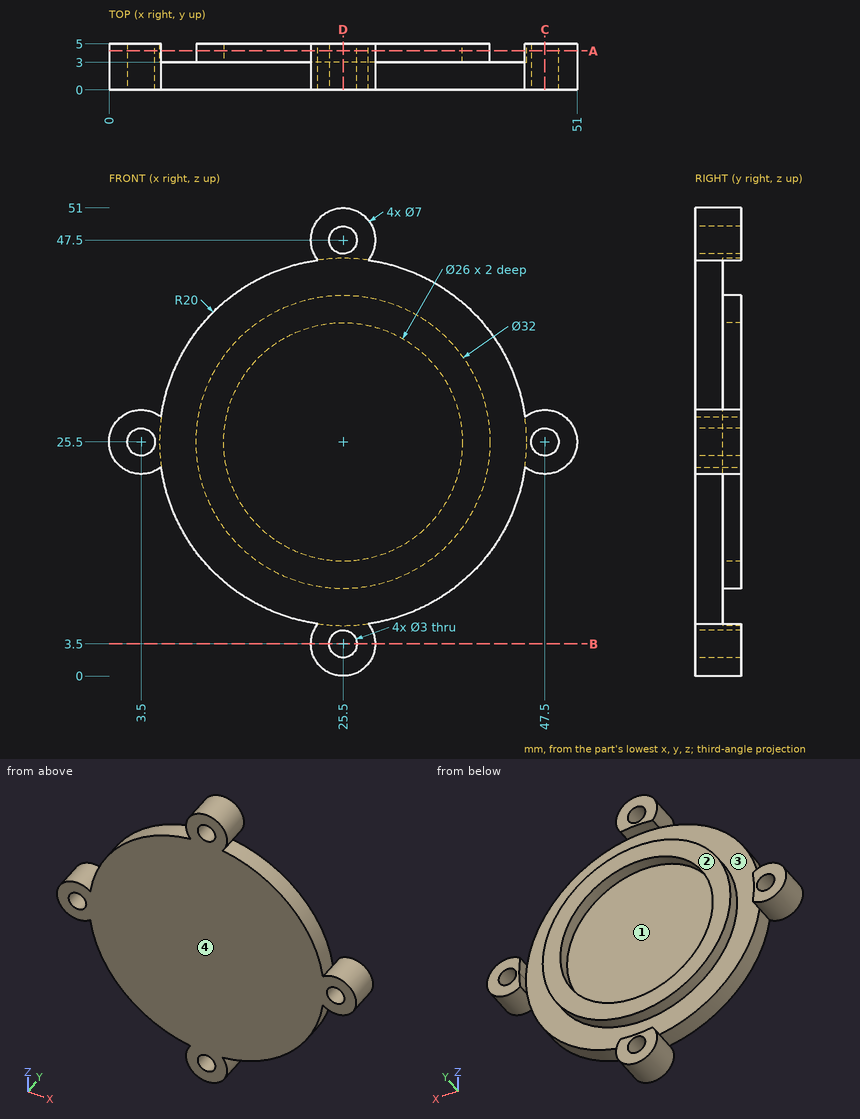
Check sheet for the drawn part. Datum: minimum x, y, z corner. Units: mm. A direction names the side the tool comes from. Round coordinates to 2 decimals unless told otherwise and drop trailing zeros. Order: outer loops, then holes, each group sorted by start corner. A loop starts at its lowest first (then second) coordinate and runs counter-clockwise, first axis right, second up. Notation, with made-up numbers: (43.5, -34) -> (101.5, -34) arc R14 cw to (101.5, -21) -> close; hole circle Ø6 at (24.5, 63.5). An arc over 180 degrees is marked (long way). Return JSON: item names as keys, results as strings. Group by question number.
Q1. Section check B-B, the plane z = 3.5. Record the boundary of the cut face in (x, y), plus the area to 3 significant figures.
Q2. Release check for a two-part mould opening along Z. For the marked faces 3 and 4 record: released by +Z, released by -Z, zero draft, split by the parting line, or undercut.
Q3. Material ranges on probe 1 along Z at (x, y) = (3.5, 3.7); probe 2 along Z at (x, y) = (24.5, 1.05), recorded low to high. Write a range as from..to.
Q4. Section check D-D, the plane x = 25.5. Record the boundary of the cut face in (y, z).
Q5. Gauge pin test, flat ends, axial feed: pin 1 (1.5 mm diameter, centred on x = 27, z = 31, fed in from +Y); pin 2 (1 mm diameter, centred on x = 43.5, y = 3, fed in from +Z); pin 3 (3 mm diameter, centred on x = 43, y = 0.5, fed in from +Z). Record the tip position at first contact, or that the pin passes through.
Q6. Tool access check on the marked faces 1 and 2. Record the directions out of +Z, -Z, +X, -X, +Y, -Y that give a thin tool (end or side, any length) a straight path to the whole face; none if there is none.
Q7. Section check A-A, the plane y = 4.25. Count the separate pieces of the cut face and the enclosed holes in it, plus the area to 3 significant figures.
Q8. Section check C-C, the plane x = 47.5. Record the boundary of the cut face in (y, z), plus the area to 3 significant figures.
Numbers:
{
 "1": {"outline": "(22, 0) -> (24, 0) -> (24, 5) -> (22, 5) -> close; (27, 0) -> (29, 0) -> (29, 5) -> (27, 5) -> close", "area": "20.0 mm^2"},
 "2": {"face 3": "undercut", "face 4": "zero draft"},
 "3": {"probe 1": "22..24, 27..29", "probe 2": "0.15..2.38, 4.62..46.38, 48.62..50.85"},
 "4": {"outline": "(0, 0) -> (5, 0) -> (5, 2) -> (0, 2) -> close; (0, 5) -> (5, 5) -> (5, 5.5) -> (3, 5.5) -> (3, 9.5) -> (5, 9.5) -> (5, 12.5) -> (3, 12.5) -> (3, 38.5) -> (5, 38.5) -> (5, 41.5) -> (3, 41.5) -> (3, 45.5) -> (5, 45.5) -> (5, 46) -> (0, 46) -> close; (0, 49) -> (5, 49) -> (5, 51) -> (0, 51) -> close"},
 "5": {"pin 1": "y = 3", "pin 2": "z = 35.18", "pin 3": "z = 37.5"},
 "6": {"face 1": "+Y", "face 2": "+Z, -Z, +X, -X, +Y"},
 "7": {"separate pieces": "5", "enclosed holes": "5", "area": "376 mm^2"},
 "8": {"outline": "(0, 22) -> (5, 22) -> (5, 24) -> (0, 24) -> close; (0, 27) -> (5, 27) -> (5, 29) -> (0, 29) -> close", "area": "20.0 mm^2"}
}
